```python
from build123d import *

# Parameters (mm, degrees)
F0_R     = 4.445
F0_R_2   = 4.826
F1_DEPTH = 3.175


with BuildPart() as f1:
    # F0 (on Top) → F1 (new body)
    with BuildSketch(Plane.XY):
        with BuildLine():
            Line((-63.881, 553.8978), (-171.831, 553.8978))
            ThreePointArc((-171.831, 553.8978), (-157.911603, 548.132197), (-152.146, 534.2128))
            ThreePointArc((-152.146, 534.2128), (-176.957475, 515.207052), (-188.845871, 544.111962))
            Line((-188.845871, 544.111962), (-230.1748, 473.075))
            Line((-230.1748, 473.075), (-255.163822, 281.038792))
            ThreePointArc((-255.163822, 281.038792), (-241.748886, 292.073428), (-229.87, 279.4))
            ThreePointArc((-229.87, 279.4), (-241.533898, 266.742335), (-255.100944, 277.334704))
            Line((-255.100944, 277.334704), (-212.279225, 17.518903))
            ThreePointArc((-212.279225, 17.518903), (-194.922014, 39.750575), (-174.1805, 20.6375))
            ThreePointArc((-174.1805, 20.6375), (-179.848602, 7.026218), (-193.502293, 1.461047))
            Line((-193.502293, 1.461047), (0, 0))
            Line((0, 0), (158.75, 0))
            ThreePointArc((158.75, 0), (186.139747, 1.581448), (213.165464, 6.304773))
            ThreePointArc((213.165464, 6.304773), (203.640017, 27.9319), (225.5393, 19.05))
            ThreePointArc((225.5393, 19.05), (224.747937, 14.627924), (222.472079, 10.754749))
            Line((222.472079, 10.754749), (253.855569, 47.390713))
            ThreePointArc((253.855569, 47.390713), (232.76785, 58.830401), (256.692111, 57.044866))
            Line((256.692111, 57.044866), (222.55606, 305.04815))
            ThreePointArc((222.55606, 305.04815), (222.650328, 304.132476), (222.6818, 303.2125))
            ThreePointArc((222.6818, 303.2125), (195.853277, 301.612028), (222.301246, 306.390742))
            Line((222.301246, 306.390742), (165.806349, 538.920196))
            ThreePointArc((165.806349, 538.920196), (166.228586, 536.583311), (166.37, 534.2128))
            ThreePointArc((166.37, 534.2128), (132.110556, 520.338774), (147.062251, 554.141805))
            Line((147.062251, 554.141805), (0, 558.8))
            Line((0, 558.8), (-25.4, 558.8))
            ThreePointArc((-25.4, 558.8), (-44.485002, 555.128282), (-63.881, 553.8978))
        make_face()
        with BuildLine():
            ThreePointArc((-174.1805, 20.6375), (-194.922014, 39.750575), (-212.279225, 17.518903))
            ThreePointArc((-212.279225, 17.518903), (-205.821316, 6.063186), (-193.502293, 1.461047))
            ThreePointArc((-193.502293, 1.461047), (-179.848602, 7.026218), (-174.1805, 20.6375))
        make_face()
        with Locations((-193.3575, 20.6375)):
            Circle(F0_R, mode=Mode.SUBTRACT)
        with BuildLine():
            ThreePointArc((-229.87, 279.4), (-241.748886, 292.073428), (-255.163822, 281.038792))
            ThreePointArc((-255.163822, 281.038792), (-255.268171, 279.184443), (-255.100944, 277.334704))
            ThreePointArc((-255.100944, 277.334704), (-241.533898, 266.742335), (-229.87, 279.4))
        make_face()
        with Locations((-242.57, 279.4)):
            Circle(F0_R, mode=Mode.SUBTRACT)
        with BuildLine():
            ThreePointArc((222.55606, 305.04815), (222.4457, 305.722682), (222.301246, 306.390742))
            ThreePointArc((222.301246, 306.390742), (195.853277, 301.612028), (222.6818, 303.2125))
            ThreePointArc((222.6818, 303.2125), (222.650328, 304.132476), (222.55606, 305.04815))
        make_face()
        with Locations((209.2198, 303.2125)):
            Circle(F0_R, mode=Mode.SUBTRACT)
        with BuildLine():
            ThreePointArc((256.8067, 55.372), (256.778019, 56.210393), (256.692111, 57.044866))
            ThreePointArc((256.692111, 57.044866), (232.76785, 58.830401), (253.855569, 47.390713))
            ThreePointArc((253.855569, 47.390713), (256.045289, 51.117293), (256.8067, 55.372))
        make_face()
        with Locations((244.5385, 55.372)):
            Circle(F0_R_2, mode=Mode.SUBTRACT)
        with BuildLine():
            ThreePointArc((225.5393, 19.05), (203.640017, 27.9319), (213.165464, 6.304773))
            ThreePointArc((213.165464, 6.304773), (218.288882, 7.546579), (222.472079, 10.754749))
            ThreePointArc((222.472079, 10.754749), (224.747937, 14.627924), (225.5393, 19.05))
        make_face()
        with Locations((212.7885, 19.05)):
            Circle(F0_R_2, mode=Mode.SUBTRACT)
        with BuildLine():
            ThreePointArc((165.806349, 538.920196), (159.000421, 549.690958), (147.062251, 554.141805))
            ThreePointArc((147.062251, 554.141805), (132.110556, 520.338774), (166.37, 534.2128))
            ThreePointArc((166.37, 534.2128), (166.228586, 536.583311), (165.806349, 538.920196))
        make_face()
        with Locations((146.431, 534.2128)):
            Circle(F0_R, mode=Mode.SUBTRACT)
        with BuildLine():
            ThreePointArc((-152.146, 534.2128), (-157.911603, 548.132197), (-171.831, 553.8978))
            ThreePointArc((-171.831, 553.8978), (-181.645128, 551.276859), (-188.845871, 544.111962))
            ThreePointArc((-188.845871, 544.111962), (-176.957475, 515.207052), (-152.146, 534.2128))
        make_face()
        with BuildLine():
            ThreePointArc((-171.831, 538.6578), (-168.68791, 537.35589), (-167.386, 534.2128))
            ThreePointArc((-167.386, 534.2128), (-174.97409, 531.06971), (-171.831, 538.6578))
        make_face(mode=Mode.SUBTRACT)
    extrude(amount=F1_DEPTH)


solid = f1.part
```
Model file for the job. Use its own axes, mm. Round coordinates to 2 decimals unless told otherwise and drop trailing zeros. Order: outer loops, then holes, each group sorted by start corner. A loop starts at its lowest first (then second) coordinate and runs counter-clockwise, first axis right, second up. Notation, with made-up numbers: (-32, -15) -> (0, -15) arc R21 cw to (0, 23) -> close; hole circle Ø5 at (60, -24.75). An arc over 180 degrees is marked (long way). Use one line per item in the form item = value.
Item 1: Drill centre lines: line 1 (Y direction, x = -14.5, z = 0.85); line 2 (X direction, y = 442, z = 0.7); line 3 (Y direction, x = -180, z = 1.7). Where is each one in solid material? Low to high.
Returned:
line_1 = 0.11 to 558.8
line_2 = -234.22 to 189.35
line_3 = 1.36 to 552.12
Item 2: Cut at C-C, the plane y = 420. Write the cut outline in (x, z) (3 decimals), and give its area (3 significant figures).
Returned:
outline = (-237.081, 0) -> (194.699, 0) -> (194.699, 3.175) -> (-237.081, 3.175) -> close
area = 1,370 mm^2
Item 3: Flat gauge pin, fed straight in: pin 1 Ø7.5 at (x, y) = (244.54, 55.37) entering from -Z. Where does the tip first touch, or does it go through?
Returned:
pin_1 = through
Item 4: Cut at A-A, the plane z = 0.6. Give the number of separate pieces and of enclosed holes in the cut face, and give its area (3 significant figures).
Returned:
separate_pieces = 1
enclosed_holes = 7
area = 249,000 mm^2
Item 5: Cut at B-B, the plane x = -220. Write the cut outline in (y, z) (3 decimals).
Returned:
outline = (64.364, 0) -> (490.564, 0) -> (490.564, 3.175) -> (64.364, 3.175) -> close
